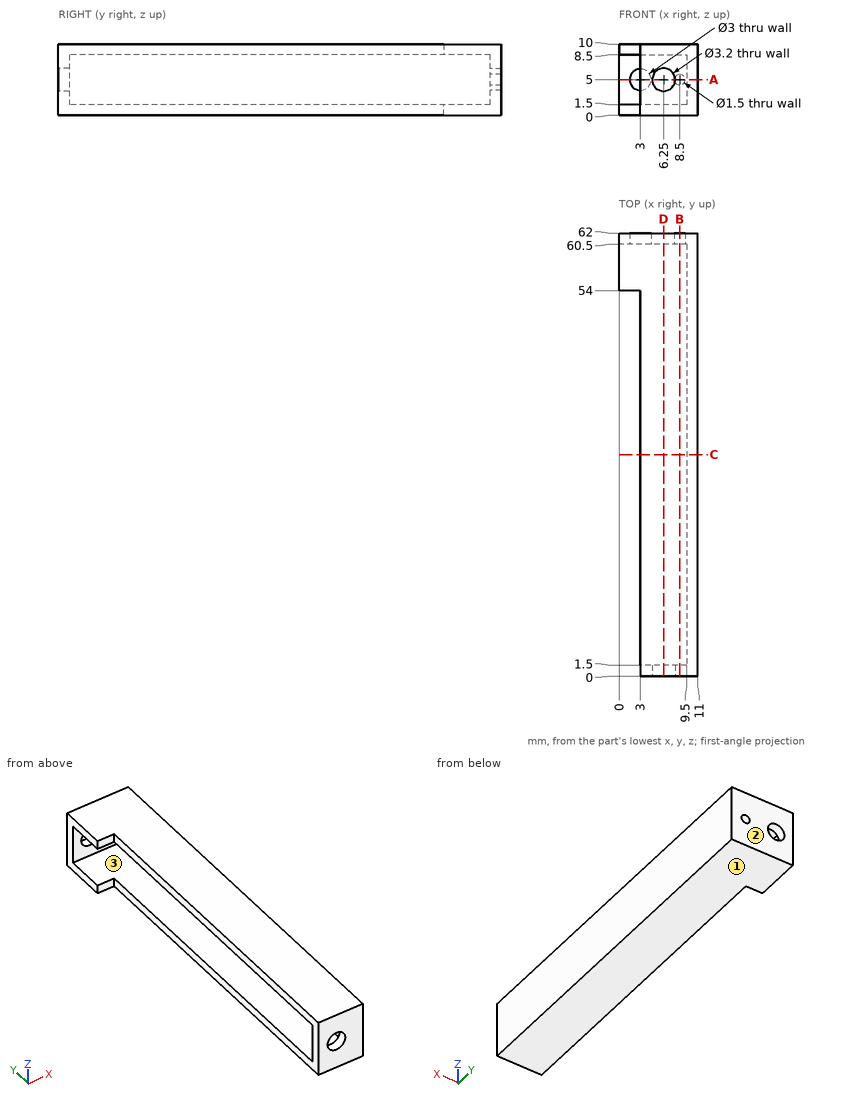
Study the drawing (mm; zero at the part's minimum x, y, z) and answer. Give positions to 0.01 mm unless a question says otherwise; leave off trailing zeros. Order: outer loops, then holes, each group sorted by start corner. A loop starts at its lowest first (then second) coordinate and runs counter-clockwise, first axis right, second up. Notation, with made-up numbers: (24.25, -10.5) -> (78.25, -10.5) arc R7 cw to (78.25, -5.5) -> close; hole circle Ø6 at (32.5, -1). An arc over 180 degrees is marked (long way). Put each result on its own line as item: value.
Item 1: Straight lines are drawn through the part: line 1 (X direction, y = 61.25, z = 5); line 2 (Z direction, x = 8.5, y = 61.1); line 3 (Z direction, x = 6.25, y = 0.35). For each, find the intervals that lie inside material, in ascending order.
Established:
line 1: x = 0 to 1.5, 4.5 to 7.75, 9.25 to 11
line 2: z = 0 to 4.25, 5.75 to 10
line 3: z = 0 to 3.4, 6.6 to 10
Item 2: A cutting plane is placed at C-C on y = 31. Give the vertices of the cut face in (x, z).
Established:
outline: (3, 0) -> (11, 0) -> (11, 10) -> (3, 10) -> (3, 8.5) -> (9.5, 8.5) -> (9.5, 1.5) -> (3, 1.5) -> close
Item 3: Given P1, Ø0.8, axis at x = 2, z = 9, coming from the -Y side; P2, Ø1, axis at y = 44.5, z = 4.5, coming from the -X side; P3, Ø5.5, axis at y = 28.5, z = 3.5, coming from the -X side, each flat-ended and moving along its own axis, determine where each tip first touches the part or whether it passes through.
Established:
P1: stops at y = 54
P2: stops at x = 9.5
P3: stops at x = 3
Item 4: For a pull along Y with two mould halves and no side action, classify the marked faces 1, 2 and 3 as released by +Y, released by -Y, zero draft, split by the parting line, or undercut.
Established:
face 1: zero draft
face 2: released by +Y
face 3: undercut
Item 5: A cutting plane is placed at A-A on z = 5. Give the vertices of the cut face in (x, y).
Established:
outline: (0, 60.5) -> (1.5, 60.5) -> (1.5, 62) -> (0, 62) -> close; (3, 0) -> (4.65, 0) -> (4.65, 1.5) -> (3, 1.5) -> close; (4.5, 60.5) -> (7.75, 60.5) -> (7.75, 62) -> (4.5, 62) -> close; (7.85, 0) -> (11, 0) -> (11, 62) -> (9.25, 62) -> (9.25, 60.5) -> (9.5, 60.5) -> (9.5, 1.5) -> (7.85, 1.5) -> close
Item 6: A cutting plane is placed at B-B on x = 8.5. Give the vertices of the cut face in (y, z).
Established:
outline: (0, 0) -> (62, 0) -> (62, 4.25) -> (60.5, 4.25) -> (60.5, 1.5) -> (1.5, 1.5) -> (1.5, 8.5) -> (60.5, 8.5) -> (60.5, 5.75) -> (62, 5.75) -> (62, 10) -> (0, 10) -> close
Item 7: A cutting plane is placed at D-D on x = 6.25. Give the vertices of the cut face in (y, z), plus the area to 3 significant figures.
Established:
outline: (0, 0) -> (62, 0) -> (62, 10) -> (0, 10) -> (0, 6.6) -> (1.5, 6.6) -> (1.5, 8.5) -> (60.5, 8.5) -> (60.5, 1.5) -> (1.5, 1.5) -> (1.5, 3.4) -> (0, 3.4) -> close
area: 202 mm^2
